```python
from build123d import *

# Parameters (mm, degrees)
SKETCH3_R           = 5
BOSS_EXTRUDE1_DEPTH = 5
SKETCH4_R           = 2.975
BOSS_EXTRUDE2_DEPTH = 10
BOSS_EXTRUDE5_DEPTH = 7.5
FILLET5_R           = 2
FILLET6_R           = 2


with BuildPart() as part:
    # Sketch3 → Boss-Extrude1 (new body)
    with BuildSketch(Plane(origin=(0, 0, 0), x_dir=(1, 0, 0), z_dir=(0, 1, 0))):
        with Locations(Location((0, 0, 0), (0, 0, 270))):
            Circle(SKETCH3_R)
    extrude(amount=BOSS_EXTRUDE1_DEPTH)

    # Sketch4 → Boss-Extrude2 (add)
    with BuildSketch(Plane(origin=(0, 5, 0), x_dir=(1, 0, 0), z_dir=(0, 1, 0))):
        with Locations(Location((0, 0, 0), (0, 0, 270))):
            Circle(SKETCH4_R)
    extrude(amount=BOSS_EXTRUDE2_DEPTH)

    # Sketch8 → Boss-Extrude5 (add, symmetric)
    with BuildSketch(Plane.XY):
        with BuildLine():
            Line((-15.5, -25), (15.5, -25))
            ThreePointArc((15.5, -25), (16.914213562, -24.414213562), (17.5, -23))
            Line((17.5, -23), (17.5, -9.571067812))
            ThreePointArc((17.5, -9.571067812), (17.119397663, -7.65765065), (16.035533906, -6.035533906))
            Line((16.035533906, -6.035533906), (11.464466094, -1.464466094))
            ThreePointArc((11.464466094, -1.464466094), (9.84234935, -0.380602337), (7.928932188, 0))
            Line((7.928932188, 0), (-7.928932188, 0))
            ThreePointArc((-7.928932188, 0), (-9.84234935, -0.380602337), (-11.464466094, -1.464466094))
            Line((-11.464466094, -1.464466094), (-16.035533906, -6.035533906))
            ThreePointArc((-16.035533906, -6.035533906), (-17.119397663, -7.65765065), (-17.5, -9.571067812))
            Line((-17.5, -9.571067812), (-17.5, -23))
            ThreePointArc((-17.5, -23), (-16.914213562, -24.414213562), (-15.5, -25))
        make_face()
        with BuildLine():
            Line((-12.5, -15.742640687), (-12.5, -18))
            ThreePointArc((-12.5, -18), (-11.914213562, -19.414213562), (-10.5, -20))
            Line((-10.5, -20), (10.5, -20))
            ThreePointArc((10.5, -20), (11.914213562, -19.414213562), (12.5, -18))
            Line((12.5, -18), (12.5, -15.742640687))
            ThreePointArc((12.5, -15.742640687), (12.271638598, -14.59459039), (11.621320344, -13.621320344))
            Line((11.621320344, -13.621320344), (2.121320344, -4.121320344))
            ThreePointArc((2.121320344, -4.121320344), (0, -3.242640687), (-2.121320344, -4.121320344))
            Line((-2.121320344, -4.121320344), (-11.621320344, -13.621320344))
            ThreePointArc((-11.621320344, -13.621320344), (-12.271638598, -14.59459039), (-12.5, -15.742640687))
        make_face(mode=Mode.SUBTRACT)
    extrude(amount=BOSS_EXTRUDE5_DEPTH, both=True)

    # Fillet5
    fillet5_edges = [part.edges().sort_by_distance(p)[0] for p in [
        (0, 0, -5),
    ]]
    fillet(fillet5_edges, radius=FILLET5_R)

    # Fillet6
    fillet6_edges = [part.edges().sort_by_distance(p)[0] for p in [
        (6.871320344, -8.871320344, -7.5),
        (0, -3.242640687, -7.5),
        (-6.871320344, -8.871320344, -7.5),
        (-12.271638598, -14.59459039, -7.5),
        (-12.5, -16.871320344, -7.5),
        (-11.914213562, -19.414213562, -7.5),
        (0, -20, -7.5),
        (11.914213562, -19.414213562, -7.5),
        (12.5, -16.871320344, -7.5),
        (12.271638598, -14.59459039, -7.5),
        (0, -3.242640687, 7.5),
        (-6.871320344, -8.871320344, 7.5),
        (-12.271638598, -14.59459039, 7.5),
        (-12.5, -16.871320344, 7.5),
        (-11.914213562, -19.414213562, 7.5),
        (0, -20, 7.5),
        (11.914213562, -19.414213562, 7.5),
        (12.5, -16.871320344, 7.5),
        (12.271638598, -14.59459039, 7.5),
        (6.871320344, -8.871320344, 7.5),
    ]]
    fillet(fillet6_edges, radius=FILLET6_R)


solid = part.part
```
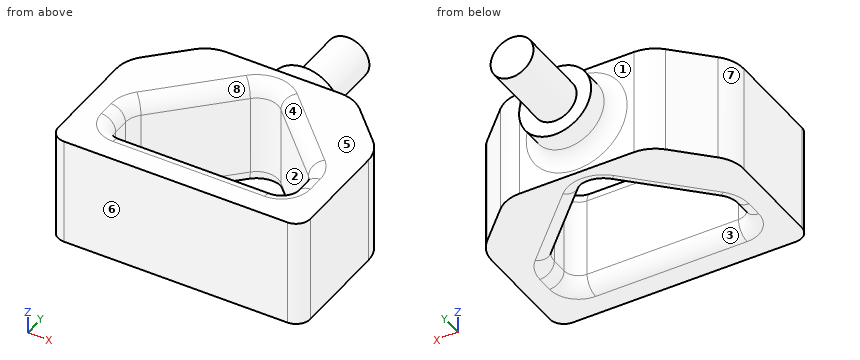
Source: CAD feature listing. Evaluate the final solid. Frame: model axes, mm. Face numbers are marked on the shaded views. A direction names the side the tool comes from. Round coordinates to 2 decimals unless told otherwise and drop trailing zeros. Loops run counter-clockwise (first coordinate to the right, second up) from the corner with the lowest first, then second, coordinate; pieces in that order, holes last.
(1) Pull-direction query (Y, two-part tool) for the marked faces 5, 6, 7 and 8; classes: +Y half, -Y half, draft (parallel to the pull), parting line (faces both ways), or undercut.
From the geometry:
face 5: draft
face 6: -Y half
face 7: +Y half
face 8: undercut
(2) Access query for the marked faces 1, 2, 3 and 4. Directions: +Z, -Z, +X, -X, +Y, -Y. A direction counts if a zero-diameter tool reaches every point of the face in a straight line with its end or side. Return the directions, or none.
From the geometry:
face 1: +Y
face 2: +Z, -Z
face 3: -Z
face 4: +Z
(3) Section query C-C (y = 8). Output: boundary loops of the cut face in (x, z) (3 decimals), and give its area (3 significant figures).
From the geometry:
outline: circle Ø5.95 at (0, 0)
area: 27.8 mm2
(4) Section query A-A (x = 0). Output: boundary loops of the cut face in (y, z) (3 decimals).
From the geometry:
outline: (-25, -7.5) - (-22, -7.5) arc R2 ccw to (-20, -5.5) - (-20, 5.5) arc R2 ccw to (-22, 7.5) - (-25, 7.5) - close; (-3.243, -5.5) arc R2 ccw to (-1.243, -7.5) - (0, -7.5) - (0, -7) arc R2 cw to (2, -5) - (5, -5) - (5, -2.975) - (15, -2.975) - (15, 2.975) - (5, 2.975) - (5, 5) - (2, 5) arc R2 cw to (0, 7) - (0, 7.5) - (-1.243, 7.5) arc R2 ccw to (-3.243, 5.5) - close
(5) Section query D-D (x = 15). Output: boundary loops of the cut face in (y, z).
From the geometry:
outline: (-25, -7.5) - (-5, -7.5) - (-5, 7.5) - (-25, 7.5) - close
(6) Contact query for flat-ended pins moving along their axis: pin 1 Ø4 at (x, z) = (-6.5, -5.5) entering from +Y; pin 2 Ø1 at (x, z) = (-7, -1) entering from +Y; pin 3 Ø8 at (y, z) = (10, -1.5) entering from +X (3 decimals). Output: stop coordinate, or through.
From the geometry:
pin 1: stops at y = 0.06
pin 2: stops at y = 0.05
pin 3: stops at x = 2.975
(7) Material intervals for probe 1 along X at (y, z) = (-17, 6.75); probe 2 along Y at (x, z) = (-7.5, -2.25); probe 3 along Y at (x, z) = (-2, -6.5), sorted ascending.
From the geometry:
probe 1: x = -17.5 to -12.94, 12.94 to 17.5
probe 2: y = -25 to -20, -9.5 to 0
probe 3: y = -25 to -20.27, -3.66 to 0.01
